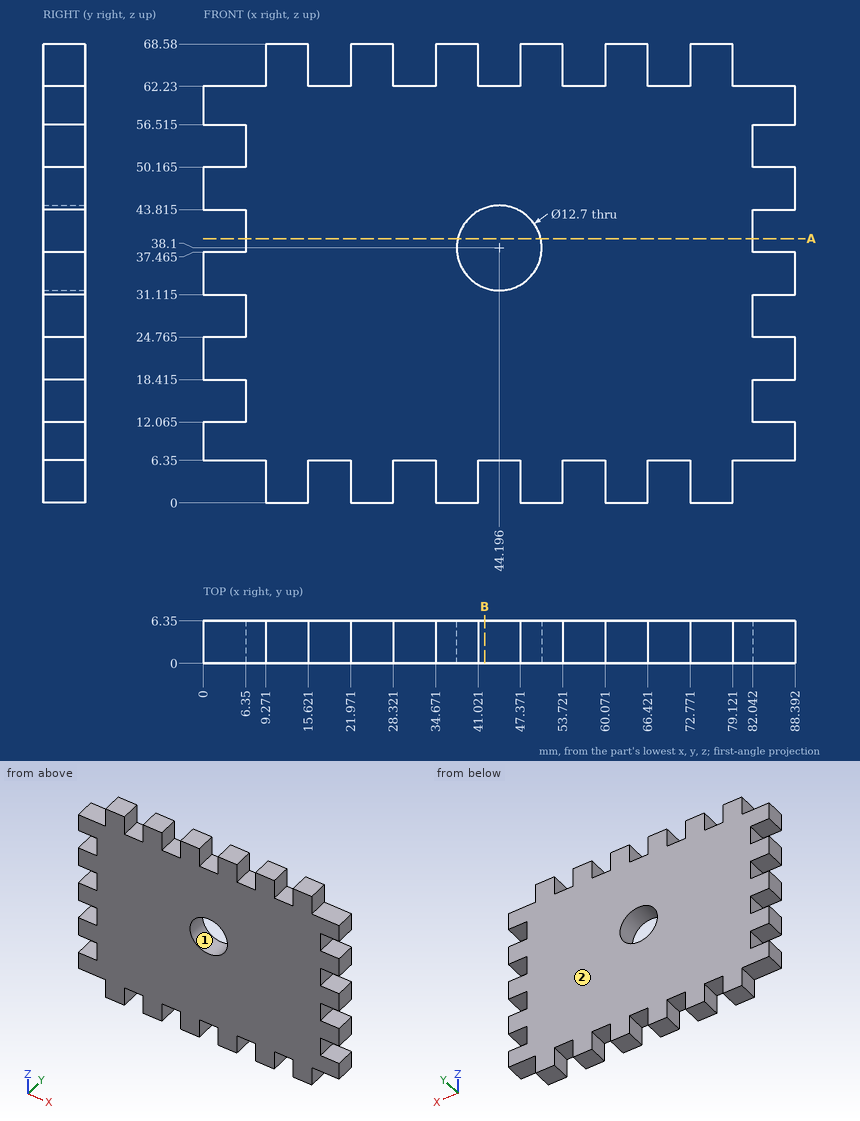
Answer from the drawing. Dimensions are ordinates in mm from the lowest x, y and z of the part. Coordinates: 2 decimals unless noted, no trailing zeros. Loops run counter-clockwise (first coordinate to the right, second up) from the corner with the lowest first, then second, coordinate; pieces in that order, holes last. Notation, with made-up numbers: (46.5, -20.5) -> (65.5, -20.5) arc R21 cw to (65.5, 1.5) -> close; hole circle Ø1 at (40, 74.25). An arc over 180 degrees is marked (long way). Answer in a Markdown table with one row per item.
Item 1: For a pull along Z with two mould halves and no side action, classify the marked faces 1 and 2 as released by +Z, released by -Z, zero draft, split by the parting line, or undercut.
Returned:
| item | result |
|---|---|
| face 1 | undercut |
| face 2 | zero draft |
Item 2: A cutting plane is placed at A-A on z = 39.5. Determine the outline of the cut face in (x, y).
Returned:
| item | result |
|---|---|
| outline | (6.35, 0) -> (38, 0) -> (38, 6.35) -> (6.35, 6.35) -> close; (50.39, 0) -> (82.04, 0) -> (82.04, 6.35) -> (50.39, 6.35) -> close |
Item 3: Straight lines are drawn through the part: line 1 along Z through (x, y) = (5, 1.75) (3 decimals); line 2 along X through (y, z) = (4, 63); line 3 along Z through (x, y) = (43.5, 2.5). For each, find the intervals that lie inside material, in ascending order. Write a range as [from, to].
Returned:
| item | result |
|---|---|
| line 1 | z = [6.35, 12.065], [18.415, 24.765], [31.115, 37.465], [43.815, 50.165], [56.515, 62.23] |
| line 2 | x = [9.27, 15.62], [21.97, 28.32], [34.67, 41.02], [47.37, 53.72], [60.07, 66.42], [72.77, 79.12] |
| line 3 | z = [6.35, 31.79], [44.41, 62.23] |
Item 4: Each of these flat-tipped pins is pushed along its axis until it touches: P1, Ø1.9, axis at y = 3, z = 2.5, coming from the -X side; P2, Ø1.9, axis at x = 31.5, y = 4, coming from the +Z side; P3, Ø10, axis at x = 29, z = 36, coming from the -Y side; P4, Ø3, axis at y = 1.5, z = 65, coming from the +X side. Where does it stop, or does it pass through?
Returned:
| item | result |
|---|---|
| P1 | stops at x = 9.27 |
| P2 | stops at z = 62.23 |
| P3 | stops at y = 0 |
| P4 | stops at x = 79.12 |
Item 5: A cutting plane is placed at B-B on x = 42. Determine the outline of the cut face in (y, z).
Returned:
| item | result |
|---|---|
| outline | (0, 6.35) -> (6.35, 6.35) -> (6.35, 32.14) -> (0, 32.14) -> close; (0, 44.06) -> (6.35, 44.06) -> (6.35, 62.23) -> (0, 62.23) -> close |
